Design review of the part built by this model. Coordinates are the model's own, in mm. Face numbers are marked on the shaded views. A direction names the side the tool comes from. Coordinates: 2 decimals unless noted, no trailing zeros. Loops run counter-clockwise (first coordinate to the right, second up) from the corner with the lowest first, then second, coordinate; pieces in that order, holes last. Notation, with made-up numbers: (-14, 4) - (-3, 4) arc R10 ccw to (-3, 8) - close; hole circle Ø4 at (0.25, -16.75). An arc over 180 degrees is marked (long way). Return JSON: item names as keys, results as strings. Group by question number.
from build123d import *

# Parameters (mm, degrees)
SKETCH1_W                  = 2.5
SKETCH1_H                  = 8
BOSS_EXTRUDE1_DEPTH        = 2.5
SKETCH2_W                  = 1.5
SKETCH2_H                  = 1.5
CUT_EXTRUDE2_DEPTH         = 7
CHAMFER3_SIZE              = 0.25
LPATTERN2_COUNT            = 6
LPATTERN2_PITCH            = 2.5
CHAMFER3_OF_LPATTERN2_SIZE = 0.25


with BuildPart() as part:
    # Sketch1 → Boss-Extrude1 (new body)
    with BuildSketch(Plane.XY):
        Rectangle(SKETCH1_W, SKETCH1_H)
    boss_extrude1 = extrude(amount=BOSS_EXTRUDE1_DEPTH)

    # Sketch2 → Cut-Extrude2 (cut)
    with BuildSketch(Plane(origin=(0, 4, 0), x_dir=(1, 0, 0), z_dir=(0, 1, 0))):
        with Locations((0, -1.25)):
            Rectangle(SKETCH2_W, SKETCH2_H)
    cut_extrude2 = extrude(amount=-CUT_EXTRUDE2_DEPTH, mode=Mode.SUBTRACT)

    # Chamfer3
    chamfer3_edges = [part.edges().sort_by_distance(p)[0] for p in [
        (0, 4, 2),
        (0.75, 4, 1.25),
        (0, 4, 0.5),
        (-0.75, 4, 1.25),
    ]]
    chamfer(chamfer3_edges, length=CHAMFER3_SIZE)

    # LPattern2: Boss-Extrude1, Cut-Extrude2 ×6
    with Locations(*[(i * LPATTERN2_PITCH, 0, 0) for i in range(1, LPATTERN2_COUNT)]):
        add(boss_extrude1)
        add(cut_extrude2, mode=Mode.SUBTRACT)

    # Chamfer3 of LPattern2
    chamfer3_of_lpattern2_edges = [part.edges().sort_by_distance(p)[0] for p in [
        (2.5, 4, 2),
        (3.25, 4, 1.25),
        (2.5, 4, 0.5),
        (1.75, 4, 1.25),
        (5, 4, 2),
        (5.75, 4, 1.25),
        (5, 4, 0.5),
        (4.25, 4, 1.25),
        (7.5, 4, 2),
        (8.25, 4, 1.25),
        (7.5, 4, 0.5),
        (6.75, 4, 1.25),
        (10, 4, 2),
        (10.75, 4, 1.25),
        (10, 4, 0.5),
        (9.25, 4, 1.25),
        (12.5, 4, 2),
        (13.25, 4, 1.25),
        (12.5, 4, 0.5),
        (11.75, 4, 1.25),
    ]]
    chamfer(chamfer3_of_lpattern2_edges, length=CHAMFER3_OF_LPATTERN2_SIZE)


solid = part.part
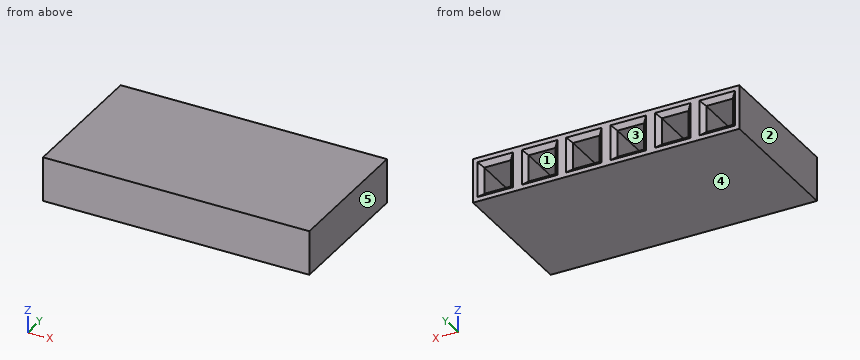
Item 1: For the marked faces 1 and 2, list the 3-axis set-ups (+Z, -Z, +X, -X, +Y, -Y) from which the entire face can be reached by the end or side of a thin tool; tool diameter is ignored.
Item 2: Draft analysis for pull direction X (two halves, no side actions). For the marked faces 3, 4 and 5, state which applies: pulls with the +X half, pulls with the -X half, needs draft (parallel to the pull), parting line crosses it, or undercut.
Item 3: Add section B-B (x = 2.5). State the section outline as (y, z) points.
Item 4: Add section A-A (y = -2.25). State the section outline as (x, z) points.
Item 5: To check wall thickness, follow line 1 (Z direction, x = 13, y = 2.25); line 2 (Y direction, x = 2, z = 1.45). State the ranges of each line that lie inside material, in increasing order. Write a range as from..to.
Item 6: For P1, Ø1.2, axis at x = 0, z = 1.5, coming from the +Y side; P2, Ø1.5, axis at x = 10, y = 3, coming from the -Z side; P3, Ø0.8, axis at x = 10, z = 1, coming from the +Y side, all flat-tipped, find the tip position at first contact; note any pin that passes through.
Answers below:
{
 "1": {"face 1": "+Y", "face 2": "+Z, -Z, -X, +Y, -Y"},
 "2": {"face 3": "undercut", "face 4": "needs draft", "face 5": "pulls with the +X half"},
 "3": {"outline": "(-4, 0) - (4, 0) - (4, 0.25) - (3.75, 0.5) - (-3, 0.5) - (-3, 2) - (3.75, 2) - (4, 2.25) - (4, 2.5) - (-4, 2.5) - close"},
 "4": {"outline": "(-1.25, 0) - (13.75, 0) - (13.75, 2.5) - (-1.25, 2.5) - close; hole (-0.75, 0.5) - (0.75, 0.5) - (0.75, 2) - (-0.75, 2) - close; hole (1.75, 0.5) - (3.25, 0.5) - (3.25, 2) - (1.75, 2) - close; hole (4.25, 0.5) - (5.75, 0.5) - (5.75, 2) - (4.25, 2) - close; hole (6.75, 0.5) - (8.25, 0.5) - (8.25, 2) - (6.75, 2) - close; hole (9.25, 0.5) - (10.75, 0.5) - (10.75, 2) - (9.25, 2) - close; hole (11.75, 0.5) - (13.25, 0.5) - (13.25, 2) - (11.75, 2) - close"},
 "5": {"line 1": "z = 0..0.5, 2..2.5", "line 2": "y = -4..-3"},
 "6": {"P1": "stops at y = 3.85", "P2": "stops at z = 0", "P3": "stops at y = -3"}
}
